Could you check a few things on this drawing? It's one solid part, dimensions in mm from its lowest x, y, z. A direction names the side the tool comes from. Coordinates: 2 decimals unless noted, no trailing zeros. Loops run counter-clockwise (first coordinate to the right, second up) from the corner with the lowest first, then second, coordinate; pieces in that order, holes last. Notation, with made-up numbers: M 84.5,13 L 133.5,13 A24 cw 133.5,50 Z; hole C 74,19.5 d4. An arc over 180 degrees is marked long. Use one line per item in the form item = value. Start each with the question number.
(1) Imagine slicing it at C-C, the plane y = 9.25. Please give me the cut outline in (x, z) (1 decimal).
(2) Will these pins go through, and if not, where does the flat tip stop? P1, Ø1.5, axis at x = 6, z = 1, coming from the -Y side; P2, Ø1.6, axis at y = 9.5, z = 2, coming from the -X side; P3, Ø0.6, axis at y = 10, z = 2, coming from the +X side.
(3) On a 3-axis mill with a long thin cutter (end or side, diameter ignored), from which of +Z, -Z, +X, -X, +Y, -Y can I reach the whole of each face in a straight line? I mean the marked faces 5 and 6. Say none if no direction works.
(4) Imagine slicing it at D-D, the plane x = 16.5. Please give me the cut outline in (y, z).
(5) Imagine slicing it at A-A, the plane x = 10. Please give me the cut outline in (y, z), and give its area (3 significant figures).
(6) Please list where these lines run through material, in increasing order: L1, parallel to Y at x = 10, z = 3.8; L2, parallel to X at y = 10.5, z = 3.4; L3, parallel to Y at x = 2, z = 3.7.
(7) Thinking about a two-plate mould opening in X: for the marked faces 1, 2, 3 and 4, which applies, +X half, -X half, draft (parallel to the pull), parting line (faces both ways), or undercut?
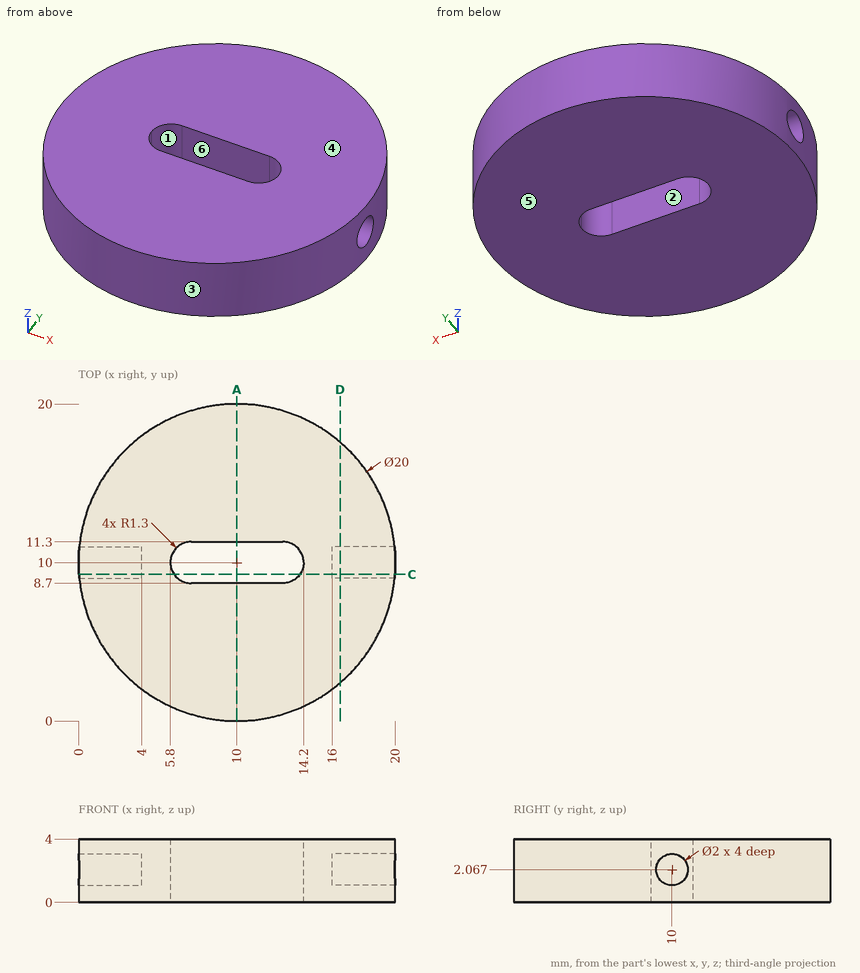
Answer:
q1.outline = M 0,0 L 6,0 L 6,4 L 0,4 L 0,2.7 L 4,2.7 L 4,1.4 L 0,1.4 Z; M 14,0 L 20,0 L 20,1.4 L 16,1.4 L 16,2.7 L 20,2.7 L 20,4 L 14,4 Z
q2.P1 = 0.54
q2.P2 = 0.01
q2.P3 = 16
q3.face_5 = -Z, +X, -X, +Y, -Y
q3.face_6 = +Z, -Z
q4.outline = M 2.4,0 L 17.6,0 L 17.6,4 L 2.4,4 Z; hole C 10,2.07 d2
q5.outline = M 0,0 L 8.7,0 L 8.7,4 L 0,4 Z; M 11.3,0 L 20,0 L 20,4 L 11.3,4 Z
q5.area = 69.6 mm²
q6.L1 = 0 to 8.7, 11.3 to 20
q6.L2 = 0.01 to 5.9, 14.1 to 19.99
q6.L3 = 4 to 16
q7.face_1 = undercut
q7.face_2 = undercut
q7.face_3 = parting line
q7.face_4 = draft
